Design review of the part built by this model. Coordinates are the model's own, in mm. Round coordinates to 2 decimals unless told otherwise and drop trailing zeros. Write each loop counter-clockwise with the first axis right and the second up, starting at its lowest first coordinate (ties: lowest second). Pieces come first, ordered by that corner, then holes.
from build123d import *

# Parameters (mm, degrees)
SKETCH1_W           = 94.5
SKETCH1_H           = 70
BOSS_EXTRUDE1_DEPTH = 3
SKETCH3_R           = 1.5
CUT_EXTRUDE2_DEPTH  = 59.877521177
FILLET2_R           = 3
SKETCH5_W           = 64
SKETCH5_H           = 56
SKETCH5_W_2         = 21.5
SKETCH5_H_2         = 18
SKETCH5_W_3         = 17.5
SKETCH5_H_3         = 15
CUT_EXTRUDE3_DEPTH  = 59.877521177
FILLET3_R           = 3


with BuildPart() as part:
    # Sketch1 → Boss-Extrude1 (new body)
    with BuildSketch(Plane(origin=(0, 0, 0), x_dir=(1, 0, 0), z_dir=(0, 1, 0))):
        Rectangle(SKETCH1_W, SKETCH1_H)
    extrude(amount=BOSS_EXTRUDE1_DEPTH)

    # Sketch3 → Cut-Extrude2 (cut, through all)
    with BuildSketch(Plane(origin=(0, 3, 0), x_dir=(1, 0, 0), z_dir=(0, 1, 0))):
        with Locations(Location((43.75, 31.5, 0), (0, 0, 270))):
            Circle(SKETCH3_R)
        with Locations(Location((-43.25, 31.5, 0), (0, 0, 270))):
            Circle(SKETCH3_R)
        with Locations(Location((-43.25, -31.5, 0), (0, 0, 270))):
            Circle(SKETCH3_R)
        with Locations(Location((43.75, -31.5, 0), (0, 0, 270))):
            Circle(SKETCH3_R)
    extrude(amount=-CUT_EXTRUDE2_DEPTH, mode=Mode.SUBTRACT)

    # Fillet2
    fillet2_edges = [part.edges().sort_by_distance(p)[0] for p in [
        (47.25, 1.5, 35),
        (-47.25, 1.5, 35),
        (-47.25, 1.5, -35),
        (47.25, 1.5, -35),
    ]]
    fillet(fillet2_edges, radius=FILLET2_R)

    # Sketch5 → Cut-Extrude3 (cut, through all)
    with BuildSketch(Plane(origin=(0, 3, 0), x_dir=(1, 0, 0), z_dir=(0, 1, 0))):
        with Locations((-8.25, 1)):
            Rectangle(SKETCH5_W, SKETCH5_H)
        with Locations((36.5, 18)):
            Rectangle(SKETCH5_W_2, SKETCH5_H_2)
        with Locations((38.5, -1.5)):
            Rectangle(SKETCH5_W_3, SKETCH5_H_3)
        with Locations((38.5, -19.5)):
            Rectangle(SKETCH5_W_3, SKETCH5_H_3)
    extrude(amount=-CUT_EXTRUDE3_DEPTH, mode=Mode.SUBTRACT)

    # Fillet3
    fillet3_edges = [part.edges().sort_by_distance(p)[0] for p in [
        (-40.25, 1.5, 27),
        (-40.25, 1.5, -29),
        (23.75, 1.5, -29),
        (23.75, 1.5, 27),
    ]]
    fillet(fillet3_edges, radius=FILLET3_R)


solid = part.part
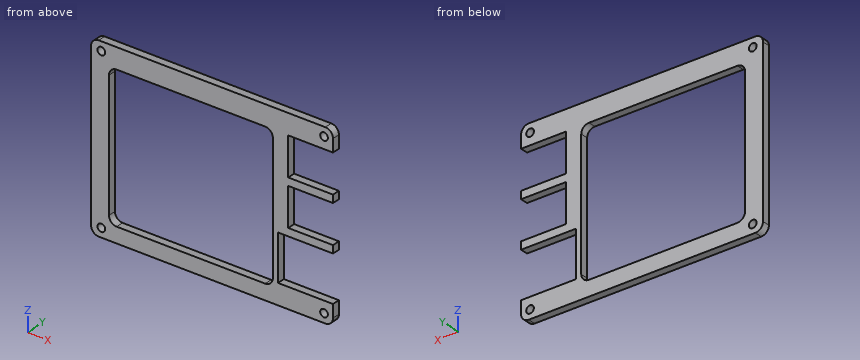
1) Add section C-C on y = 0.85. Count the separate pieces of the cut face and the enclosed holes in it, and give its area (3 significant figures).
2) Add section A-A on z = -17. State the section outline as (x, y) points, and give its area (3 significant figures).
3) Add section B-B on x = -36. State the section outline as (y, z) points.
4) For line 1 along X through (y, z) = (1.35, -31.5); line 2 along Z through (x, y) = (31, 0.6); line 3 along X through (y, z) = (2.15, -2.5), list the stretches that pass through material, from the lowest coordinate up.
5) For P1, Ø1.5, axis at y = 1.5, z = -14, coming from the +X side; P2, Ø1.5, axis at y = 1, z = 20.5, coming from the +X side, all flat-tipped, find the tip position at first contact; note any pin that passes through.
Computed:
1. separate pieces: 1
1. enclosed holes: 5
1. area: 2,090 mm2
2. outline: (-47.25, 0) - (-40.25, 0) - (-40.25, 3) - (-47.25, 3) - close; (23.75, 0) - (25.75, 0) - (25.75, 3) - (23.75, 3) - close
2. area: 27.0 mm2
3. outline: (0, -35) - (3, -35) - (3, -29) - (0, -29) - close; (0, 27) - (3, 27) - (3, 35) - (0, 35) - close
4. line 1: x = -47.25 to -44.75, -41.75 to 42.25, 45.25 to 47.25
4. line 2: z = -35 to -27, -9 to -6, 9 to 12, 27 to 35
4. line 3: x = -47.25 to -40.25, 23.75 to 29.75
5. P1: stops at x = 25.75
5. P2: stops at x = 29.75
